Model file for the job. Use its own axes, mm. Face numbers are marked on the shaded views. A direction names the side the tool comes from. Round coordinates to 2 decimals unless told otherwise and drop trailing zeros. Loops run counter-clockwise (first coordinate to the right, second up) from the corner with the lowest first, then second, coordinate; pieces in that order, holes last. Notation, with made-up numbers: (73, -37) - (104, -37) arc R12 ccw to (104, -28) - close; hole circle Ø5 at (12, 2). An arc over 180 degrees is marked (long way). Answer as a JSON object with one key per item and string values.
from build123d import *

# Parameters (mm, degrees)
SKETCH1_W             = 19
SKETCH1_H             = 10
BOSS_EXTRUDE1_DEPTH   = 18
SKETCH1_H_2           = 3.2
BOSS_EXTRUDE1_2_DEPTH = 18
SKETCH1_6_W           = 12.45
SKETCH1_6_H           = 3.2
BOSS_EXTRUDE6_DEPTH   = 38
BOSS_EXTRUDE7_DEPTH   = 10
SKETCH4_W             = 18
SKETCH4_H             = 10
SKETCH4_H_2           = 3.2
BOSS_EXTRUDE8_DEPTH   = 3
CUT_EXTRUDE1_START    = -10
SKETCH6_R             = 1.5
CUT_EXTRUDE1_DEPTH    = 20
BOSS_EXTRUDE10_REACH  = 45.922
SKETCH7_W             = 2
SKETCH7_H             = 38
BOSS_EXTRUDE11_REACH  = 47.95
SKETCH8_W             = 7.5
SKETCH8_H             = 3
SKETCH9_R             = 2
CUT_EXTRUDE2_DEPTH    = 2
CUT_EXTRUDE3_START    = -10.45
CUT_EXTRUDE3_DEPTH    = 8.45


# Read off the part's stored shape, not the designer's step: Cut-Extrude3
with BuildPart() as part:
    # Sketch1 → Boss-Extrude1 (new body)
    with BuildSketch(Plane.XY):
        with Locations((7.125, 0)):
            Rectangle(SKETCH1_W, SKETCH1_H)
    extrude(amount=-BOSS_EXTRUDE1_DEPTH)



with BuildPart() as body_2:
    # Sketch1 → Boss-Extrude1 2 (new body)
    with BuildSketch(Plane.XY):
        with Locations((7.125, 13.4)):
            Rectangle(SKETCH1_W, SKETCH1_H_2)
    extrude(amount=-BOSS_EXTRUDE1_2_DEPTH)


with BuildPart() as part_1:
    add(part.part)

    add(body_2.part)  # Boss-Extrude6 merges body 2
    # Sketch1<6> → Boss-Extrude6 (add)
    with BuildSketch(Plane.XY):
        Polygon((-14.825, 5), (-14.825, -2), (-9.825, -2), (-9.825, -5), (-2.375, -5), (-2.375, 5), align=None)
        with Locations((-8.6, 13.4)):
            Rectangle(SKETCH1_6_W, SKETCH1_6_H)
    extrude(amount=-BOSS_EXTRUDE6_DEPTH)

    # Sketch1<7> → Boss-Extrude7 (add)
    with BuildSketch(Plane.XY):
        Polygon((-14.825, -2), (-14.825, -3.3), (-14.825, -5), (-9.825, -5), (-9.825, -2), align=None)
    extrude(amount=-BOSS_EXTRUDE7_DEPTH)

    # Sketch4 → Boss-Extrude8 (add)
    with BuildSketch(Plane(origin=(16.625, 0, 0), x_dir=(0, 0, -1), z_dir=(1, 0, 0))):
        with Locations((9, 0)):
            Rectangle(SKETCH4_W, SKETCH4_H)
        with Locations((9, 13.4)):
            Rectangle(SKETCH4_W, SKETCH4_H_2)
    extrude(amount=BOSS_EXTRUDE8_DEPTH)

    # Sketch6 → Cut-Extrude1 (cut)
    with BuildSketch(Plane(origin=(0, 5, 0), x_dir=(1, 0, 0), z_dir=(0, 1, 0)).offset(CUT_EXTRUDE1_START)):
        with Locations(Location((10.44201924, 11.5, 0), (0, 0, 270))):
            Circle(SKETCH6_R)
    extrude(amount=CUT_EXTRUDE1_DEPTH, mode=Mode.SUBTRACT)

    # Sketch7 → Boss-Extrude10 (add, up to next)
    with BuildSketch(Plane(origin=(0, 5, 0), x_dir=(1, 0, 0), z_dir=(0, 1, 0)), mode=Mode.PRIVATE) as boss_extrude10_sk1:
        with Locations((-3.375, 19)):
            Rectangle(SKETCH7_W, SKETCH7_H)
    boss_extrude10_tool1 = extrude(boss_extrude10_sk1.sketch, amount=BOSS_EXTRUDE10_REACH, mode=Mode.PRIVATE) - part_1.part
    # Sketch7 → Boss-Extrude10 (add, up to next)
    with BuildSketch(Plane(origin=(0, 5, 0), x_dir=(1, 0, 0), z_dir=(0, 1, 0)), mode=Mode.PRIVATE) as boss_extrude10_sk2:
        with Locations((-13.825, 19)):
            Rectangle(SKETCH7_W, SKETCH7_H)
    boss_extrude10_tool2 = extrude(boss_extrude10_sk2.sketch, amount=BOSS_EXTRUDE10_REACH, mode=Mode.PRIVATE) - part_1.part
    add(boss_extrude10_tool1.solids().sort_by_distance((-3.375, 5, -19))[0])
    add(boss_extrude10_tool2.solids().sort_by_distance((-13.825, 5, -19))[0])

    # Sketch8 → Boss-Extrude11 (add, up to next)
    with BuildSketch(Plane.XZ.offset(-11.8), mode=Mode.PRIVATE) as boss_extrude11_sk1:
        with Locations((15.875, -1.5)):
            Rectangle(SKETCH8_W, SKETCH8_H)
    boss_extrude11_tool1 = extrude(boss_extrude11_sk1.sketch, amount=BOSS_EXTRUDE11_REACH, mode=Mode.PRIVATE) - part_1.part
    add(boss_extrude11_tool1.solids().sort_by_distance((15.875, 11.8, -1.5))[0])

    # Sketch9 → Cut-Extrude2 (cut)
    with BuildSketch(Plane.ZY.offset(14.825)):
        with Locations(Location((-8.095100141, 4.609535031, 0), (0, 0, 270))):
            Circle(SKETCH9_R)
    extrude(amount=-CUT_EXTRUDE2_DEPTH, mode=Mode.SUBTRACT)

    # Cut-Extrude3 outline → Cut-Extrude3 (cut)
    with BuildSketch(Plane.ZY.offset(14.825).offset(CUT_EXTRUDE3_START)):
        with BuildLine():
            Line((-3.612072469, 5), (-15.943641317, 5))
            Line((-15.943641317, 5), (-16.601615213, 4.609535031))
            Line((-16.601615213, 4.609535031), (-9.291615213, 0.271522619))
            ThreePointArc((-9.291615213, 0.271522619), (-5.215878744, 1.151199572), (-3.612072469, 5))
        make_face()
    extrude(amount=CUT_EXTRUDE3_DEPTH, mode=Mode.SUBTRACT)


solid = part_1.part
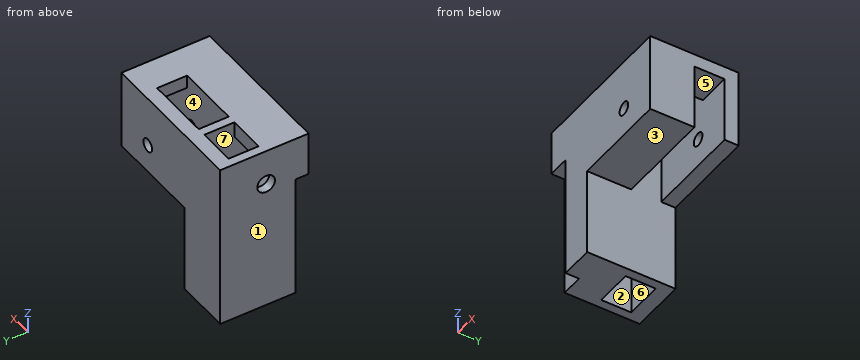
1) Slice it at A-A on x = -9. List the corners of the cut face in (y, z).
Values follow:
{"outline": "(-5, -38) - (5, -38) - (5, -15.94) - (4.61, -16.6) - (0.27, -9.29) arc R4.5 cw to (5, -3.61) - (5, 0) - (-5, 0) - close; (11.8, -38) - (15, -38) - (15, 0) - (11.8, 0) - close"}
2) Probe probe 1 along Y at (x, z) = (2.5, -17); probe 2 along X at (y, z) = (5.25, -21) (3 decimals); probe 3 along X at (y, z) = (-3, -11.5) (3 decimals). List the from-to ranges inside material, lowest first.
Values follow:
{"probe 1": "-5 to 5, 11.8 to 15", "probe 2": "-14.825 to -12.825, -4.375 to -2.375", "probe 3": "-9.825 to 8.942, 11.942 to 19.625"}
3) Two-plate mould, pull along X, no slides. Class the marked faces 1, 2 and 3: pulls with the +X half, pulls with the -X half, needs draft (parallel to the pull), parting line crosses it, or undercut.
Values follow:
{"face 1": "pulls with the -X half", "face 2": "undercut", "face 3": "needs draft"}
4) Slice it at C-C on z = -11.5. List the corners of the cut face in (x, y) (3 decimals).
Values follow:
{"outline": "(-14.825, -2) - (-9.825, -2) - (-9.825, -5) - (8.942, -5) - (8.942, 5) - (-2.375, 5) - (-2.375, 11.8) - (8.942, 11.8) - (8.942, 15) - (-14.825, 15) - close; (11.942, -5) - (19.625, -5) - (19.625, 5) - (11.942, 5) - close; (11.942, 11.8) - (19.625, 11.8) - (19.625, 15) - (11.942, 15) - close; hole (-12.825, 1.582) - (-4.375, 1.582) - (-4.375, 11.8) - (-12.825, 11.8) - close"}
5) Slice it at D-D on z = -25. List the corners of the cut face in (x, y) (3 decimals).
Values follow:
{"outline": "(-14.825, -2) - (-9.825, -2) - (-9.825, -5) - (-2.375, -5) - (-2.375, 15) - (-14.825, 15) - close; hole (-12.825, 5) - (-4.375, 5) - (-4.375, 11.8) - (-12.825, 11.8) - close"}
6) Tool access for the marked faces 4, 5, 6 and 7: list every direction of +Z, -Z, +X, -X, +Y, -Y with a clear straight run to the whole face (end or side of a thin tool).
Values follow:
{"face 4": "-Z", "face 5": "-Z, +X", "face 6": "+Z, -Z", "face 7": "none"}
7) Slice it at B-B on y = 9.25. List the corners of the cut face in (x, z) (3 decimals), then the cut area to 4 significant figures.
Values follow:
{"outline": "(-14.825, -38) - (-12.825, -38) - (-12.825, 0) - (-14.825, 0) - close; (-4.375, -38) - (-2.375, -38) - (-2.375, 0) - (-4.375, 0) - close; (12.125, -3) - (19.625, -3) - (19.625, 0) - (12.125, 0) - close", "area": "174.5 mm²"}
8) Drop flat-ended pins along their axis: P1, Ø6, axis at x = 9.5, y = -1.5, coming from the -Z side; P2, Ø2.5, axis at x = -13.5, z = -22, coming from the -Y side; P3, Ø0.9, axis at x = -13, y = -3.5, coming from the -Z side. Give the stop position or say it passes through.
Values follow:
{"P1": "z = -18", "P2": "y = -2", "P3": "z = -10"}
